from build123d import *

# Parameters (mm, degrees)
BOSS_EXTRUDE1_DEPTH = 300
FILLET1_R           = 1
FILLET2_R           = 0.3
SKETCH3_W           = 0.4
SKETCH3_H           = 0.6
CUT_EXTRUDE1_DEPTH  = 300
FILLET3_R           = 0.4


with BuildPart() as part:
    # Sketch1 → Boss-Extrude1 (new body)
    with BuildSketch(Plane.XY):
        with BuildLine():
            Line((-3.9, 0), (3.9, 0))
            Line((3.9, 0), (3.9, 1.6))
            Line((3.9, 1.6), (3.3, 1.6))
            ThreePointArc((3.3, 1.6), (2.8, 2.1), (3.3, 2.6))
            Line((3.3, 2.6), (4.3, 2.6))
            Line((4.3, 2.6), (4.3, 3.2))
            Line((4.3, 3.2), (9.6, 3.2))
            Line((9.6, 3.2), (9.6, 0.2))
            Line((9.6, 0.2), (11, 0.2))
            Line((11, 0.2), (11, -6.730696291))
            Line((11, -6.730696291), (7.88474386, -7.28))
            Line((7.88474386, -7.28), (7.88474386, -14.32))
            Line((7.88474386, -14.32), (11, -14.869303709))
            Line((11, -14.869303709), (11, -20.4))
            Line((11, -20.4), (9.8, -20.4))
            ThreePointArc((9.8, -20.4), (9.517157288, -20.517157288), (9.4, -20.8))
            Line((9.4, -20.8), (9.4, -41.8))
            ThreePointArc((9.4, -41.8), (8.9, -42.3), (8.4, -41.8))
            Line((8.4, -41.8), (8.4, -20.8))
            ThreePointArc((8.4, -20.8), (8.282842712, -20.517157288), (8, -20.4))
            Line((8, -20.4), (4.5, -20.4))
            ThreePointArc((4.5, -20.4), (4, -19.9), (4.5, -19.4))
            Line((4.5, -19.4), (8.4, -19.4))
            Line((8.4, -19.4), (9.6, -19.4))
            ThreePointArc((9.6, -19.4), (9.882842712, -19.282842712), (10, -19))
            Line((10, -19), (10, -15.70840334))
            Line((10, -15.70840334), (6.88474386, -15.159099631))
            Line((6.88474386, -15.159099631), (6.88474386, -11.2))
            ThreePointArc((6.88474386, -11.2), (6.767586572, -10.917157288), (6.48474386, -10.8))
            Line((6.48474386, -10.8), (-6.48474386, -10.8))
            ThreePointArc((-6.48474386, -10.8), (-6.767586572, -10.917157288), (-6.88474386, -11.2))
            Line((-6.88474386, -11.2), (-6.88474386, -15.159099631))
            Line((-6.88474386, -15.159099631), (-10, -15.70840334))
            Line((-10, -15.70840334), (-10, -19))
            ThreePointArc((-10, -19), (-9.882842712, -19.282842712), (-9.6, -19.4))
            Line((-9.6, -19.4), (-8.4, -19.4))
            Line((-8.4, -19.4), (-4.5, -19.4))
            ThreePointArc((-4.5, -19.4), (-4, -19.9), (-4.5, -20.4))
            Line((-4.5, -20.4), (-8, -20.4))
            ThreePointArc((-8, -20.4), (-8.282842712, -20.517157288), (-8.4, -20.8))
            Line((-8.4, -20.8), (-8.4, -41.8))
            ThreePointArc((-8.4, -41.8), (-8.9, -42.3), (-9.4, -41.8))
            Line((-9.4, -41.8), (-9.4, -20.8))
            ThreePointArc((-9.4, -20.8), (-9.517157288, -20.517157288), (-9.8, -20.4))
            Line((-9.8, -20.4), (-11, -20.4))
            Line((-11, -20.4), (-11, -14.869303709))
            Line((-11, -14.869303709), (-7.88474386, -14.32))
            Line((-7.88474386, -14.32), (-7.88474386, -7.28))
            Line((-7.88474386, -7.28), (-11, -6.730696291))
            Line((-11, -6.730696291), (-11, 0.2))
            Line((-11, 0.2), (-9.6, 0.2))
            Line((-9.6, 0.2), (-9.6, 3.2))
            Line((-9.6, 3.2), (-4.3, 3.2))
            Line((-4.3, 3.2), (-4.3, 2.6))
            Line((-4.3, 2.6), (-3.3, 2.6))
            ThreePointArc((-3.3, 2.6), (-2.8, 2.1), (-3.3, 1.6))
            Line((-3.3, 1.6), (-3.9, 1.6))
            Line((-3.9, 1.6), (-3.9, 0))
        make_face()
        with BuildLine():
            Line((-6.88474386, -6.440900369), (-6.88474386, -9.4))
            ThreePointArc((-6.88474386, -9.4), (-6.767586572, -9.682842712), (-6.48474386, -9.8))
            Line((-6.48474386, -9.8), (6.48474386, -9.8))
            ThreePointArc((6.48474386, -9.8), (6.767586572, -9.682842712), (6.88474386, -9.4))
            Line((6.88474386, -9.4), (6.88474386, -6.440900369))
            Line((6.88474386, -6.440900369), (10, -5.89159666))
            Line((10, -5.89159666), (10, -0.8))
            Line((10, -0.8), (8.6, -0.8))
            Line((8.6, -0.8), (8.6, 2.2))
            Line((8.6, 2.2), (5.3, 2.2))
            Line((5.3, 2.2), (5.3, 1.6))
            Line((5.3, 1.6), (4.9, 1.6))
            Line((4.9, 1.6), (4.9, -1))
            Line((4.9, -1), (-4.9, -1))
            Line((-4.9, -1), (-4.9, 1.6))
            Line((-4.9, 1.6), (-5.3, 1.6))
            Line((-5.3, 1.6), (-5.3, 2.2))
            Line((-5.3, 2.2), (-8.6, 2.2))
            Line((-8.6, 2.2), (-8.6, -0.8))
            Line((-8.6, -0.8), (-10, -0.8))
            Line((-10, -0.8), (-10, -5.89159666))
            Line((-10, -5.89159666), (-6.88474386, -6.440900369))
        make_face(mode=Mode.SUBTRACT)
    extrude(amount=BOSS_EXTRUDE1_DEPTH)

    # Fillet1
    fillet1_edges = [part.edges().sort_by_distance(p)[0] for p in [
        (4.9, -1, 150),
        (-4.9, -1, 150),
    ]]
    fillet(fillet1_edges, radius=FILLET1_R)

    # Fillet2
    fillet2_edges = [part.edges().sort_by_distance(p)[0] for p in [
        (8.6, -0.8, 150),
        (8.6, 2.2, 150),
        (-8.6, 2.2, 150),
        (-8.6, -0.8, 150),
        (-10, -0.8, 150),
    ]]
    fillet(fillet2_edges, radius=FILLET2_R)

    # Sketch3 → Cut-Extrude1 (cut)
    with BuildSketch(Plane(origin=(0, 0, 0), x_dir=(-1, 0, 0), z_dir=(0, 0, -1))):
        with Locations((5.1, 1.9)):
            Rectangle(SKETCH3_W, SKETCH3_H)
        with Locations((-5.1, 1.9)):
            Rectangle(SKETCH3_W, SKETCH3_H)
    extrude(amount=-CUT_EXTRUDE1_DEPTH, mode=Mode.SUBTRACT)

    # Fillet3
    fillet3_edges = [part.edges().sort_by_distance(p)[0] for p in [
        (-6.88474386, -6.440900369, 150),
        (6.88474386, -6.440900369, 150),
        (-4.9, 2.2, 150),
        (4.9, 2.2, 150),
    ]]
    fillet(fillet3_edges, radius=FILLET3_R)


solid = part.part
Check sheet for the modelled part. Datum: model origin and axes. Units: mm. A direction names the side the tool comes from. Round coordinates to 2 decimals unless told otherwise and drop trailing zeros. Loops run counter-clockwise (first coordinate to the right, second up) from the corner with the lowest first, then second, coordinate; pieces in that order, holes last.
1. Mould release check, pull along X, two halves, no side actions. Record for faces 5 (the flat face through (-10, -3, 148)), 6 (the flat face through (-11, -3, 148)), 7 (the flat face through (7.4, -12.7, 300)): released by +X, released by -X, zero draft, split by the parting line, or undercut.
2. Gauge pin test, flat ends, axial feed: pin 1 Ø3.5 at (y, z) = (1, 100.5) entering from -X; pin 2 Ø6.5 at (y, z) = (-33, 194.5) entering from -X; pin 3 Ø0.5 at (y, z) = (1, 224) entering from +X; pin 4 Ø6.5 at (x, z) = (3, 133.5) entering from -Y. Record the tip position at first contact, or that the pin passes through.
3. Scan lines: probe 1 along X at (y, z) = (0.5, 251); probe 2 along Y at (x, z) = (6.5, 100.5); probe 3 along Y at (x, z) = (3.5, 42). Record each from-to range of solid material in increasing order.
4. Sectioned sample at A-A on y = -28. Record the boundary of the cut face in (x, z), and give its area (3 significant figures).
5. Set-up check for faces 1 (the flat face through (8.4, -31, 148)), 2 (the flat face through (10, -3, 148)), 3 (the flat face through (-9.4, -31, 148)), 4 (the flat face through (7.885, -11, 148)): record each of +Z, -Z, +X, -X, +Y, -Y from which the full face is reachable in a straight line by a thin tool's end or side.
Recorded:
1. face 5: undercut
1. face 6: released by -X
1. face 7: zero draft
2. pin 1: stops at x = -11
2. pin 2: stops at x = -9.4
2. pin 3: stops at x = 9.6
2. pin 4: stops at y = -20.4
3. probe 1: x = -9.6 to -8.6, -4.9 to -3.9, 3.9 to 4.9, 8.6 to 9.6
3. probe 2: y = -20.4 to -19.4, -10.8 to -9.8, 2.2 to 3.2
3. probe 3: y = -10.8 to -9.8, -1 to 0, 1.6 to 2.6
4. outline: (-9.4, 0) - (-8.4, 0) - (-8.4, 300) - (-9.4, 300) - close; (8.4, 0) - (9.4, 0) - (9.4, 300) - (8.4, 300) - close
4. area: 600 mm2
5. face 1: +Z, -Z, -Y
5. face 2: +Z, -Z
5. face 3: +Z, -Z, -X, -Y
5. face 4: +Z, -Z, +X
